Could you check a few things on this drawing? It's one solid part, dimensions in mm from its lowest x, y, z. A direction names the side the tool comes from. Give positions to 0.01 mm unless a question says otherwise; leave off trailing zeros. Loops run counter-clockwise (first coordinate to the right, second up) from the corner with the lowest first, then second, coordinate; pieces in that order, holes last.
Q1. Suppose I cut it at C-C (z = 36.5). List the corners of the cut face in (x, y) for me.
Q2. For the marked faces 1, 2, 3, 4 and 5, which set-ups out of +Z, -Z, +X, -X, +Y, -Y let a thin tool reach every point of the face, with its end or its side?
Q3. Suppose I cut it at A-A (y = 35). List the corners of the cut face in (x, z) for me, and give its area (3 significant figures).
Q4. I need wall thicknesses on probe 1 along X at (y, z) = (20, 16.5); probe 2 along Z at (x, y) = (13, 47.5). Which ranges of each line are inside material? Lowest first, please.
Q5. Suppose I cut it at D-D (y = 46). List the corners of the cut face in (x, z) for me.
Q6. I'm going to push flat-ended pins straight in: P1, Ø12, axis at y = 22, z = 17, coming from the -X side; P2, Ø10, axis at y = 38.5, z = 53.5, coming from the +X side; P3, Ø5, axis at x = 10, y = 10.5, coming from the +Z side. Where does each tip first touch, or does it pass through?
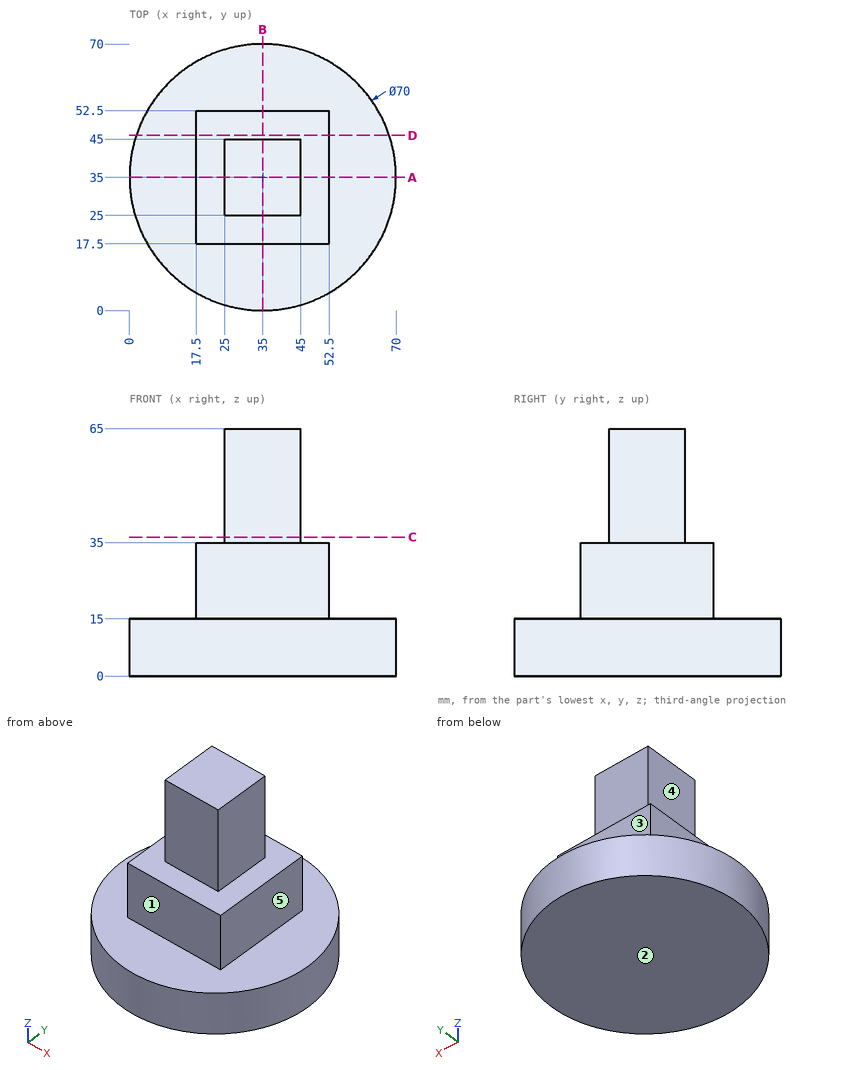
Solutions:
1. outline: (25, 25) - (45, 25) - (45, 45) - (25, 45) - close
2. face 1: +Z, +X, -X, -Y
2. face 2: -Z, +X, -X, +Y, -Y
2. face 3: +Z, +X, -X, +Y
2. face 4: +Z, -X, +Y, -Y
2. face 5: +Z, +X, +Y, -Y
3. outline: (0, 0) - (70, 0) - (70, 15) - (52.5, 15) - (52.5, 35) - (45, 35) - (45, 65) - (25, 65) - (25, 35) - (17.5, 35) - (17.5, 15) - (0, 15) - close
3. area: 2,350 mm2
4. probe 1: x = 17.5 to 52.5
4. probe 2: z = 0 to 15
5. outline: (1.77, 0) - (68.23, 0) - (68.23, 15) - (52.5, 15) - (52.5, 35) - (17.5, 35) - (17.5, 15) - (1.77, 15) - close
6. P1: stops at x = 0.78
6. P2: stops at x = 45
6. P3: stops at z = 15
